For this review, take the finished solid that the model builds, in its own axes (mm). A direction names the side the tool comes from. Coordinates: 2 decimals unless noted, no trailing zeros. Write each loop counter-clockwise with the first axis right and the second up, starting at its lowest first coordinate (ties: lowest second). Pieces come first, ordered by that corner, then holes.
1) We need section A-A on z = 13. Write out the cut boundary in (x, y), then the cut area to 3 significant figures.
2) For faces 5 (the face through (-10, 17, -10)), 6 (the face through (0, 0, 3)), 7 (the face through (0, -12, 23)), 8 (the face through (-10.59, 21.78, -3.41)), list the 3-axis set-ups (+Z, -Z, +X, -X, +Y, -Y) from which the entire face can be reached by the end or side of a thin tool; tool diameter is ignored.
3) Mouldability with a two-part tool opening along Y and no side actions: class faces 1 (the face through (0, 10.25, 23)), 2 (the face through (0, 17.32, 1)), 3 (the face through (-13.57, -20.06, -3.41)), 4 (the face through (0, -17.32, 1)) as pulls with the +Y half, pulls with the -Y half, needs draft (parallel to the pull), parting line crosses it, or undercut.
4) We need section B-B on x = 0. Write out the cut boundary in (y, z).
5) We need section C-C on y = -1. Write out the cut boundary in (x, z), then the cut area to 3 significant figures.
6) Insertion check: P1, Ø2, axis at x = 5.5, y = -1.5, coming from the +Z side; P2, Ø9, axis at y = 0, z = 37, coming from the -X side; P3, Ø2, axis at x = 13, y = 8.5, coming from the -Z side; P4, Ø22.5, axis at x = -2, y = 3, coming from the +Z side. Each pin has a flat end and moves straight along its axis. Give the tip position at first contact, or say it passes through.
7) To check wall thickness, follow line 1 along Y through (x, z) = (-2.5, 10); line 2 along Z through (x, y) = (0, 11.65); line 3 along X through (y, z) = (-4, 2.5). State the ranges of each line that lie inside material, in increasing order.
8) We need section D-D on z = 37. Write out the cut boundary in (x, y), then the cut area to 3 significant figures.
Autodesk Fusion 360 part; units mm, degrees
sketch "Sketch1" plane through (0, 0, 0) normal (0, 0, 1) x (1, 0, 0)
  circle A0 centre (0, 0) radius 5
  line L0 (10, 17.3205) -> (-10, 17.3205)
  line L1 (-10, 17.3205) -> (-20, 0)
  line L2 (-20, 0) -> (-10, -17.3205)
  line L3 (-10, -17.3205) -> (10, -17.3205)
  line L4 (10, -17.3205) -> (20, 0)
  line L5 (20, 0) -> (10, 17.3205)
  circle A1 centre (10, 17.3205) radius 4.5
  circle A2 centre (20, 0) radius 4.5
  circle A3 centre (10, -17.3205) radius 4.5
  circle A4 centre (-10, -17.3205) radius 4.5
  circle A5 centre (-20, 0) radius 4.5
  circle A6 centre (-10, 17.3205) radius 4.5
  dimension "d1" = 10
  dimension "d2" = 20
  dimension "d3" = 9
  dimension "d4" = 9
  dimension "d5" = 9
  dimension "d6" = 9
  dimension "d7" = 9
  dimension "d8" = 9
extrude "Extrude1" add sketch "Sketch1" against normal blind 10 contours A0 | L0 L1 A6 | L0 L1 A6 | L0 L5 A1 | L0 L5 A1 | L1 L2 A5 | L1 L2 A5 | L4 L5 A2 | L4 L5 A2 | L2 L3 A4 | L2 L3 A4 | L3 L4 A3 | L3 L4 A3 makes body 1 at (-5.5224, 17.7686, -3.3333) makes body 2 at (14.4776, -16.8725, -3.3333) makes body 3 at (14.4776, 17.7686, -3.3333) makes body 4 at (-15.5224, 0.4481, -3.3333) makes body 5 at (-5.5224, -16.8725, -3.3333) makes body 6 at (24.4944, -0.2243, -6.6667) makes body 7 at (4.9938, -0.2492, -6.6667)
extrude "Extrude2" add sketch "Sketch1" along normal blind 3 contours A0 | L0 L1 A6 | L0 L1 A6 | L0 L1 L2 L3 L4 L5 A1 A2 A3 A4 A5 A6 | L0 L5 A1 | L0 L5 A1 | L1 L2 A5 | L1 L2 A5 | L4 L5 A2 | L4 L5 A2 | L2 L3 A4 | L2 L3 A4 | L3 L4 A3 | L3 L4 A3 bodies 1 7 2 3 4 5 6
sketch "Sketch2" plane through (0, 0, 3) normal (0, 0, 1) x (1, 0, 0)
  line L0 (10.25, -10.25) -> (-10.25, -10.25)
  line L1 (-10.25, -10.25) -> (-10.25, 10.25)
  line L2 (-10.25, 10.25) -> (10.25, 10.25)
  line L3 (10.25, 10.25) -> (10.25, -10.25)
  line L4 (10.25, -10.25) -> (-10.25, 10.25) construction
  line L5 (-10.25, -10.25) -> (10.25, 10.25) construction
  line L6 (12, -12) -> (-12, -12)
  line L7 (-12, -12) -> (-12, 12)
  line L8 (-12, 12) -> (12, 12)
  line L9 (12, 12) -> (12, -12)
  line L10 (12, -12) -> (-12, 12) construction
  line L11 (-12, -12) -> (12, 12) construction
  arc A0 (-5.5, 17.3205) -> (-12.25, 13.4234) centre (-10, 17.3205) ccw
  line L12 (-12.25, 13.4234) -> (-17.75, 3.8971)
  arc A1 (-17.75, 3.8971) -> (-17.75, -3.8971) centre (-20, 0) ccw
  line L13 (-17.75, -3.8971) -> (-12.25, -13.4234)
  arc A2 (-12.25, -13.4234) -> (-5.5, -17.3205) centre (-10, -17.3205) ccw
  line L14 (-5.5, -17.3205) -> (5.5, -17.3205)
  arc A3 (5.5, -17.3205) -> (12.25, -13.4234) centre (10, -17.3205) ccw
  line L15 (12.25, -13.4234) -> (17.75, -3.8971)
  arc A4 (17.75, -3.8971) -> (17.75, 3.8971) centre (20, 0) ccw
  line L16 (17.75, 3.8971) -> (12.25, 13.4234)
  arc A5 (12.25, 13.4234) -> (5.5, 17.3205) centre (10, 17.3205) ccw
  line L17 (5.5, 17.3205) -> (-5.5, 17.3205)
  dimension "d13" = 20.5
  dimension "d14" = 20.5
  dimension "d15" = 24
  dimension "d16" = 24
extrude "Extrude3" add sketch "Sketch2" along normal blind 40 contours L6 L7 L8 L9 bodies 1
sketch "Sketch3" plane through (12, 0, 0) normal (1, 0, 0) x (0, 1, 0)
  line L0 (-12, 3) -> (12, 3)
  line L1 (12, 3) -> (12, 43)
  line L2 (12, 43) -> (-12, 43)
  line L3 (-12, 43) -> (-12, 3)
  circle A0 centre (0, 37) radius 2.75
  dimension "d19" = 5.5
extrude "Extrude4" cut sketch "Sketch3" against normal blind 31 contours A0 bodies 1
pattern_circular "C-Pattern1" count 4 over 360 about axis through (0, 0, 1.75) along (0, 0, 1) of "Extrude4"
Result:
1. outline: (-12, -12) - (12, -12) - (12, 12) - (-12, 12) - close; hole (-10.25, -10.25) - (10.25, -10.25) - (10.25, 10.25) - (-10.25, 10.25) - close
1. area: 156 mm2
2. face 5: -Z, +X, -X, +Y, -Y
2. face 6: +Z
2. face 7: +Z, +X, -X, -Y
2. face 8: -Z
3. face 1: undercut
3. face 2: pulls with the +Y half
3. face 3: undercut
3. face 4: pulls with the -Y half
4. outline: (-17.32, 0) - (-5, 0) - (-5, -10) - (5, -10) - (5, 0) - (17.32, 0) - (17.32, 3) - (12, 3) - (12, 34.25) - (10.25, 34.25) - (10.25, 3) - (-10.25, 3) - (-10.25, 34.25) - (-12, 34.25) - (-12, 3) - (-17.32, 3) - close; (-12, 39.75) - (-10.25, 39.75) - (-10.25, 43) - (-12, 43) - close; (10.25, 39.75) - (12, 39.75) - (12, 43) - (10.25, 43) - close
5. outline: (-24.39, -10) - (-15.61, -10) - (-15.61, 0) - (-4.9, 0) - (-4.9, -10) - (4.9, -10) - (4.9, 0) - (15.61, 0) - (15.61, -10) - (24.39, -10) - (24.39, 3) - (12, 3) - (12, 34.44) - (10.25, 34.44) - (10.25, 3) - (-10.25, 3) - (-10.25, 34.44) - (-12, 34.44) - (-12, 3) - (-24.39, 3) - close; (-12, 39.56) - (-10.25, 39.56) - (-10.25, 43) - (-12, 43) - close; (10.25, 39.56) - (12, 39.56) - (12, 43) - (10.25, 43) - close
5. area: 542 mm2
6. P1: stops at z = 3
6. P2: stops at x = -12
6. P3: stops at z = 0
6. P4: stops at z = 43
7. line 1: y = -12 to -10.25, 10.25 to 12
7. line 2: z = 0 to 34.25, 39.75 to 43
7. line 3: x = -22.06 to -17.94, -17.69 to 17.69, 17.94 to 22.06
8. outline: (-12, -12) - (-2.75, -12) - (-2.75, -10.25) - (-10.25, -10.25) - (-10.25, -2.75) - (-12, -2.75) - close; (-12, 2.75) - (-10.25, 2.75) - (-10.25, 10.25) - (-2.75, 10.25) - (-2.75, 12) - (-12, 12) - close; (2.75, -12) - (12, -12) - (12, -2.75) - (10.25, -2.75) - (10.25, -10.25) - (2.75, -10.25) - close; (2.75, 10.25) - (10.25, 10.25) - (10.25, 2.75) - (12, 2.75) - (12, 12) - (2.75, 12) - close
8. area: 117 mm2
